Geometry: final body of the model. Coordinates: model frame, mm. Round coordinates to 2 decimals unless told otherwise and drop trailing zeros. Loops run counter-clockwise (first coordinate to the right, second up) from the corner with the lowest first, then second, coordinate; pieces in that order, holes last. Notation, with made-up numbers: (85.5, 86) -> (137.5, 86) arc R26 ccw to (137.5, 109) -> close; hole circle Ø4 at (29.5, 55). An arc over 180 degrees is marked (long way). Answer in a Markdown table with one row per item.
```python
from build123d import *

# Parameters (mm, degrees)
BOSS_EXTRUDE1_DEPTH = 4.08
CUT_EXTRUDE1_DEPTH  = 0.3


with BuildPart() as part:
    # Sketch1 → Boss-Extrude1 (new body)
    with BuildSketch(Plane(origin=(0, 0, 0), x_dir=(1, 0, 0), z_dir=(0, 1, 0))):
        with BuildLine():
            Line((0.15, 0), (0.15, 0.512520873))
            Line((0.15, 0.512520873), (-6.232557616, 2.372866767))
            ThreePointArc((-6.232557616, 2.372866767), (-8.110196222, 5.002527571), (-11.041610225, 3.643316544))
            Line((-11.041610225, 3.643316544), (-10.770722466, 3.514398655))
            ThreePointArc((-10.770722466, 3.514398655), (-8.071596063, 4.67869548), (-6.561988987, 2.156403483))
            Line((-6.561988987, 2.156403483), (-0.15, 0.287479127))
            Line((-0.15, 0.287479127), (-0.15, 0))
            Line((-0.15, 0), (0.15, 0))
        make_face()
    extrude(amount=BOSS_EXTRUDE1_DEPTH)

    # Sketch2 → Cut-Extrude1 (cut)
    with BuildSketch(Plane(origin=(0.149434274, 0, -0.512685767), x_dir=(-0.9600498543859307, 0, -0.27982901403098553), z_dir=(0.27982901403098553, 0, -0.9600498543859307))):
        with BuildLine():
            Line((0.97346461, 1.39), (0.97346461, 2.69))
            Line((0.97346461, 2.69), (5.47346461, 2.69))
            ThreePointArc((5.47346461, 2.69), (6.12346461, 2.04), (5.47346461, 1.39))
            Line((5.47346461, 1.39), (0.97346461, 1.39))
        make_face()
    extrude(amount=-CUT_EXTRUDE1_DEPTH, mode=Mode.SUBTRACT)


solid = part.part
```
Item 1: Cut plane D-D (y = 0.55). Output: boundary loops of the cut face in (x, z).
Answer:
| item | result |
|---|---|
| outline | (-11.04, -3.64) arc R2.53 ccw to (-6.23, -2.37) -> (0.15, -0.51) -> (0.15, 0) -> (-0.15, 0) -> (-0.15, -0.29) -> (-6.56, -2.16) arc R2.23 cw to (-10.77, -3.51) -> close |
Item 2: Cut plane A-A (z = -1.3). Output: boundary loops of the cut face in (x, y), then the cut area to 3 significant figures.
Answer:
| item | result |
|---|---|
| outline | (-3.62, 0) -> (-2.55, 0) -> (-2.55, 1.39) -> (-3.62, 1.39) -> close; (-3.62, 2.69) -> (-2.55, 2.69) -> (-2.55, 4.08) -> (-3.62, 4.08) -> close |
| area | 2.98 mm² |
Item 3: Line query: probe 1 along X at (y, z) = (2.3, -4.5); probe 2 along Z at (x, y) = (-7, 1.2); probe 3 along Z at (x, y) = (-7.5, 1.3). Output: solid intervals per line, ascending. Write a range as [from, to].
Answer:
| item | result |
|---|---|
| probe 1 | x = [-10.38, -9.85], [-7.66, -7.14] |
| probe 2 | z = [-4.38, -3.93] |
| probe 3 | z = [-4.75, -4.4] |
Item 4: Cut plane C-C (y = 1.75). Output: boundary loops of the cut face in (x, z).
Answer:
| item | result |
|---|---|
| outline | (-11.04, -3.64) arc R2.53 ccw to (-6.23, -2.37) -> (-5.66, -2.21) -> (-5.75, -1.92) -> (-6.56, -2.16) arc R2.23 cw to (-10.77, -3.51) -> close; (-0.87, -0.5) -> (-0.79, -0.79) -> (0.15, -0.51) -> (0.15, 0) -> (-0.15, 0) -> (-0.15, -0.29) -> close |
Item 5: Pin query (flat end, axial travel): pin 1 Ø2 at (x, y) = (-6.5, 2.5) entering from -Z. Return the tip coordinate at first contact, or that it passes through.
Answer:
| item | result |
|---|---|
| pin 1 | stops at z = -4.75 |
Item 6: Cut plane B-B (x = -3). Output: boundary loops of the cut face in (y, z).
Answer:
| item | result |
|---|---|
| outline | (0, -1.43) -> (1.39, -1.43) -> (1.39, -1.12) -> (0, -1.12) -> close; (2.69, -1.43) -> (4.08, -1.43) -> (4.08, -1.12) -> (2.69, -1.12) -> close |
